Could you check a few things on this model? Use its own coordinates, in mm. A direction names the side the tool comes from. Coordinates: 2 decimals unless noted, no trailing zeros. Write each loop counter-clockwise with the first axis right and the second up, starting at its lowest first coordinate (ties: lowest second). Pieces come first, ordered by that corner, then holes.
```python
from build123d import *

# Parameters (mm, degrees)
F0_W     = 68.8
F0_H     = 53.5
F1_DEPTH = 25
F2_R     = 1.6
F3_DEPTH = 25
F4_W     = 12
F4_H     = 10.8
F5_DEPTH = 6.6
F6_W     = 8.8
F6_H     = 10.8
F7_DEPTH = 2


with BuildPart() as f1:
    # F0 (on Top) → F1 (new body)
    with BuildSketch(Plane.XY):
        Rectangle(F0_W, F0_H)
    extrude(amount=F1_DEPTH)

    # F2 (on face) → F3 (cut)
    with BuildSketch(Plane.XY.offset(25)):
        with Locations((-19, 24.25)):
            Circle(F2_R)
        with Locations((31.9, 8.75)):
            Circle(F2_R)
        with Locations((-20.4, -24.25)):
            Circle(F2_R)
        with Locations((31.9, -19.15)):
            Circle(F2_R)
    extrude(amount=-F3_DEPTH, mode=Mode.SUBTRACT)

    # F4 (on face) → F5 (join)
    with BuildSketch(Plane(origin=(-34.4, 0, 0), x_dir=(0, -1, 0), z_dir=(-1, 0, 0))):
        with Locations((-11.35, 8.7)):
            Rectangle(F4_W, F4_H)
    extrude(amount=F5_DEPTH)

    # F6 (on face) → F7 (join)
    with BuildSketch(Plane(origin=(-34.4, 0, 0), x_dir=(0, -1, 0), z_dir=(-1, 0, 0))):
        with Locations((18.15, 9.176207)):
            Rectangle(F6_W, F6_H)
    extrude(amount=F7_DEPTH)


solid = f1.part
```
1. I want a section at B-B on z = 16.25. Please give me the cut outline in (x, y).
Verdict:
outline: (-34.4, -26.75) - (34.4, -26.75) - (34.4, 26.75) - (-34.4, 26.75) - close; hole circle Ø3.2 at (-20.4, -24.25); hole circle Ø3.2 at (-19, 24.25); hole circle Ø3.2 at (31.9, -19.15); hole circle Ø3.2 at (31.9, 8.75)
2. I want a section at C-C on x = 31.9. Please give me the cut outline in (y, z).
Verdict:
outline: (-26.75, 0) - (-20.75, 0) - (-20.75, 25) - (-26.75, 25) - close; (-17.55, 0) - (7.15, 0) - (7.15, 25) - (-17.55, 25) - close; (10.35, 0) - (26.75, 0) - (26.75, 25) - (10.35, 25) - close
3. I want a section at A-A on y = 8.75. Please give me the cut outline in (x, z), plus the area to 3 significant figures.
Verdict:
outline: (-41, 3.3) - (-34.4, 3.3) - (-34.4, 0) - (30.3, 0) - (30.3, 25) - (-34.4, 25) - (-34.4, 14.1) - (-41, 14.1) - close; (33.5, 0) - (34.4, 0) - (34.4, 25) - (33.5, 25) - close
area: 1,710 mm2
4. Please list where these lines run through material, in increasing order: line 1 along Y through (x, z) = (31.9, 17.5); line 2 along Y through (x, z) = (-20.4, 10.5); line 3 along X through (y, z) = (1, 18.75).
Verdict:
line 1: y = -26.75 to -20.75, -17.55 to 7.15, 10.35 to 26.75
line 2: y = -26.75 to -25.85, -22.65 to 23.48, 25.02 to 26.75
line 3: x = -34.4 to 34.4
5. I want a section at D-D on y = 16. Please give me the cut outline in (x, z), plus the area to 3 significant figures.
Verdict:
outline: (-41, 3.3) - (-34.4, 3.3) - (-34.4, 0) - (34.4, 0) - (34.4, 25) - (-34.4, 25) - (-34.4, 14.1) - (-41, 14.1) - close
area: 1,790 mm2
6. For pin 1 (0.6 mm diameter, centred on x = -35.5, y = -19, fed in from +Z); pin 2 (2 mm diameter, centred on x = -35.5, z = 10.5, fed in from -Y); pin 3 (10 mm diameter, centred on y = -21, z = 8.5, fed in from -X), each with a flat end and sliding along its axis, tell me the tip position at first contact or that it passes through.
Verdict:
pin 1: stops at z = 14.58
pin 2: stops at y = -22.55
pin 3: stops at x = -36.4
7. On a 3-axis mill with a long thin cutter (end or side, diameter ignored), from which of +Z, -Z, +X, -X, +Y, -Y can I reach the whole of each face in a straight line? I mean faces 4 (the face through (-35, -18, 14.576)), 5 (the face through (-35, -18, 3.776)), 6 (the face through (-38, 5.35, 9)). Say none if no direction works.
Verdict:
face 4: +Z, -X, +Y, -Y
face 5: -Z, -X, -Y
face 6: +Z, -Z, -X
8. If we mould it in two halves opening along X, with no side actions, what happens to faces 1 (the face through (-36.4, -18, 9)), 2 (the face through (-21.58, -23.17, 12.68)), 3 (the face through (-38, 11, 3.3))? For each: pulls with the +X half, pulls with the -X half, needs draft (parallel to the pull), parting line crosses it, or undercut.
Verdict:
face 1: pulls with the -X half
face 2: undercut
face 3: needs draft
